For this review, take the finished solid that the model builds, in its own axes (mm). A direction names the side the tool comes from. Give positions to 0.01 mm unless a question says otherwise; leave off trailing zeros. Write each loop counter-clockwise with the first axis right and the second up, starting at its lowest first coordinate (ties: lowest second). Pieces come first, ordered by that corner, then holes.
Q1. We need section B-B (y = 122.5). Write out the cut boundary in (x, z), then the cut area to 3 significant figures.
Q2. For line 1 (X direction, y = 31, z = 0.75) (3 decimals); line 2 (X direction, y = 74, z = 6.25) (3 decimals); line 3 (X direction, y = 91, z = 0.5), list the stretches that pass through material, from the lowest coordinate up.
Q3. We need section A-A (y = 44.45). Write out the cut boundary in (x, z) (3 decimals).
Q4. Insertion check: P1, Ø3, axis at y = 33, z = 3, coming from the +X side; P2, Ø3, axis at x = 83, z = 3.5, coming from the -Y side; P3, Ø1.9, axis at y = 24.5, z = 4.5, coming from the +X side. Each pin has a flat end and moves straight along its axis. Give the tip position at first contact, or say it passes through.
Q5. Machinability: for faces 1 (the flat face through (-2, -12, 6.35)), 2 (the flat face through (38.1, 5, 3)), 3 (the flat face through (51, 28.448, 3)), which of the approach directions +Z, -Z, +X, -X, +Y, -Y give a long, thin tool a straight path to every point of the face, cutting with its end or side? Answer none if there is none.
Q6. Mouldability with a two-part tool opening along X and no side actions: class faces 4 (the flat face through (-2, -12, 0)), 5 (the cylindrical face through (-5.04, -82.45, 3.13)), 6 (the flat face through (-38.1, 5, 3)) as released by +X, released by -X, zero draft, split by the parting line, or undercut.
Q7. We need section D-D (x = 27.5). Write out the cut boundary in (y, z), then the cut area to 3 significant figures.
Q8. We need section C-C (x = 0). Write out the cut boundary in (y, z).
```python
from build123d import *

# Parameters (mm, degrees)
BOSS_EXTRUDE1_DEPTH = 6.35
CUT_EXTRUDE1_REACH  = 210.789
SKETCH2_R           = 1.3335
SKETCH2_W           = 24.765
SKETCH2_H           = 71.755
CUT_EXTRUDE2_REACH  = 210.789
SKETCH3_R           = 0.635
CUT_EXTRUDE3_DEPTH  = 209.788828163
FILLET1_START       = -1
FILLET1_DEPTH       = 8
FILLET1_2_DEPTH     = 6.35
SKETCH5_R           = 2.0828
CUT_EXTRUDE4_DEPTH  = 209.788828163


with BuildPart() as part:
    # Sketch1 → Boss-Extrude1 (new body)
    with BuildSketch(Plane.XY):
        with BuildLine():
            Line((-38.1, 92.71), (-38.1, 165.60027858))
            ThreePointArc((-38.1, 165.60027858), (0, -82.55), (38.1, 165.60027858))
            Line((38.1, 165.60027858), (38.1, 92.71))
            Line((38.1, 92.71), (38.1, -6.35))
            Line((38.1, -6.35), (-38.1, -6.35))
            Line((-38.1, -6.35), (-38.1, 92.71))
        make_face()
    extrude(amount=BOSS_EXTRUDE1_DEPTH)

    # Sketch2 → Cut-Extrude1 (cut, up to next)
    with BuildSketch(Plane(origin=(0, 0, 0), x_dir=(-1, 0, 0), z_dir=(0, 0, -1)), mode=Mode.PRIVATE) as cut_extrude1_sk1:
        with Locations((61.7855, 12.5095)):
            Circle(SKETCH2_R)
    cut_extrude1_tool1 = extrude(cut_extrude1_sk1.sketch, amount=-CUT_EXTRUDE1_REACH, mode=Mode.PRIVATE) & part.part
    # Sketch2 → Cut-Extrude1 (cut, up to next)
    with BuildSketch(Plane(origin=(0, 0, 0), x_dir=(-1, 0, 0), z_dir=(0, 0, -1)), mode=Mode.PRIVATE) as cut_extrude1_sk2:
        with Locations((61.7855, 84.6455)):
            Circle(SKETCH2_R)
    cut_extrude1_tool2 = extrude(cut_extrude1_sk2.sketch, amount=-CUT_EXTRUDE1_REACH, mode=Mode.PRIVATE) & part.part
    # Sketch2 → Cut-Extrude1 (cut, up to next)
    with BuildSketch(Plane(origin=(0, 0, 0), x_dir=(-1, 0, 0), z_dir=(0, 0, -1)), mode=Mode.PRIVATE) as cut_extrude1_sk3:
        with Locations((89.9795, 84.6455)):
            Circle(SKETCH2_R)
    cut_extrude1_tool3 = extrude(cut_extrude1_sk3.sketch, amount=-CUT_EXTRUDE1_REACH, mode=Mode.PRIVATE) & part.part
    # Sketch2 → Cut-Extrude1 (cut, up to next)
    with BuildSketch(Plane(origin=(0, 0, 0), x_dir=(-1, 0, 0), z_dir=(0, 0, -1)), mode=Mode.PRIVATE) as cut_extrude1_sk4:
        with Locations((89.9795, 12.5095)):
            Circle(SKETCH2_R)
    cut_extrude1_tool4 = extrude(cut_extrude1_sk4.sketch, amount=-CUT_EXTRUDE1_REACH, mode=Mode.PRIVATE) & part.part
    # Sketch2 → Cut-Extrude1 (cut, up to next)
    with BuildSketch(Plane(origin=(0, 0, 0), x_dir=(-1, 0, 0), z_dir=(0, 0, -1)), mode=Mode.PRIVATE) as cut_extrude1_sk5:
        with Locations((75.8825, 48.5775)):
            Rectangle(SKETCH2_W, SKETCH2_H)
    cut_extrude1_tool5 = extrude(cut_extrude1_sk5.sketch, amount=-CUT_EXTRUDE1_REACH, mode=Mode.PRIVATE) & part.part
    add(cut_extrude1_tool1.solids().sort_by_distance((-61.7855, 12.5095, 0))[0], mode=Mode.SUBTRACT)
    add(cut_extrude1_tool2.solids().sort_by_distance((-61.7855, 84.6455, 0))[0], mode=Mode.SUBTRACT)
    add(cut_extrude1_tool3.solids().sort_by_distance((-89.9795, 84.6455, 0))[0], mode=Mode.SUBTRACT)
    add(cut_extrude1_tool4.solids().sort_by_distance((-89.9795, 12.5095, 0))[0], mode=Mode.SUBTRACT)
    add(cut_extrude1_tool5.solids().sort_by_distance((-75.8825, 48.5775, 0))[0], mode=Mode.SUBTRACT)

    # Sketch3 → Cut-Extrude2 (cut, up to next)
    with BuildSketch(Plane.XY.offset(6.35), mode=Mode.PRIVATE) as cut_extrude2_sk1:
        with Locations((-66.04, 6.35)):
            Circle(SKETCH3_R)
    cut_extrude2_tool1 = extrude(cut_extrude2_sk1.sketch, amount=-CUT_EXTRUDE2_REACH, mode=Mode.PRIVATE) & part.part
    # Sketch3 → Cut-Extrude2 (cut, up to next)
    with BuildSketch(Plane.XY.offset(6.35), mode=Mode.PRIVATE) as cut_extrude2_sk2:
        with Locations((-71.628, 6.35)):
            Circle(SKETCH3_R)
    cut_extrude2_tool2 = extrude(cut_extrude2_sk2.sketch, amount=-CUT_EXTRUDE2_REACH, mode=Mode.PRIVATE) & part.part
    # Sketch3 → Cut-Extrude2 (cut, up to next)
    with BuildSketch(Plane.XY.offset(6.35), mode=Mode.PRIVATE) as cut_extrude2_sk3:
        with Locations((-80.137, 6.35)):
            Circle(SKETCH3_R)
    cut_extrude2_tool3 = extrude(cut_extrude2_sk3.sketch, amount=-CUT_EXTRUDE2_REACH, mode=Mode.PRIVATE) & part.part
    # Sketch3 → Cut-Extrude2 (cut, up to next)
    with BuildSketch(Plane.XY.offset(6.35), mode=Mode.PRIVATE) as cut_extrude2_sk4:
        with Locations((-85.725, 6.35)):
            Circle(SKETCH3_R)
    cut_extrude2_tool4 = extrude(cut_extrude2_sk4.sketch, amount=-CUT_EXTRUDE2_REACH, mode=Mode.PRIVATE) & part.part
    # Sketch3 → Cut-Extrude2 (cut, up to next)
    with BuildSketch(Plane.XY.offset(6.35), mode=Mode.PRIVATE) as cut_extrude2_sk5:
        with Locations((-73.0885, 90.805)):
            Circle(SKETCH3_R)
    cut_extrude2_tool5 = extrude(cut_extrude2_sk5.sketch, amount=-CUT_EXTRUDE2_REACH, mode=Mode.PRIVATE) & part.part
    # Sketch3 → Cut-Extrude2 (cut, up to next)
    with BuildSketch(Plane.XY.offset(6.35), mode=Mode.PRIVATE) as cut_extrude2_sk6:
        with Locations((-78.6765, 90.805)):
            Circle(SKETCH3_R)
    cut_extrude2_tool6 = extrude(cut_extrude2_sk6.sketch, amount=-CUT_EXTRUDE2_REACH, mode=Mode.PRIVATE) & part.part
    add(cut_extrude2_tool1.solids().sort_by_distance((-66.04, 6.35, 6.35))[0], mode=Mode.SUBTRACT)
    add(cut_extrude2_tool2.solids().sort_by_distance((-71.628, 6.35, 6.35))[0], mode=Mode.SUBTRACT)
    add(cut_extrude2_tool3.solids().sort_by_distance((-80.137, 6.35, 6.35))[0], mode=Mode.SUBTRACT)
    add(cut_extrude2_tool4.solids().sort_by_distance((-85.725, 6.35, 6.35))[0], mode=Mode.SUBTRACT)
    add(cut_extrude2_tool5.solids().sort_by_distance((-73.0885, 90.805, 6.35))[0], mode=Mode.SUBTRACT)
    add(cut_extrude2_tool6.solids().sort_by_distance((-78.6765, 90.805, 6.35))[0], mode=Mode.SUBTRACT)

    # Sketch4 → Cut-Extrude3 (cut, through all)
    with BuildSketch(Plane.XY.offset(6.35)):
        Polygon((-48.26, 72.898), (-48.26, 53.848), (-58.1, 53.848), (-58.1, 28.448), (-43.18, 28.448), (-43.18, 19.558), (-38.1, 19.558), (-38.1, 72.898), align=None)
        Polygon((43.18, 28.448), (58.1, 28.448), (58.1, 53.848), (48.26, 53.848), (48.26, 72.898), (38.1, 72.898), (38.1, 19.558), (43.18, 19.558), align=None)
    extrude(amount=-CUT_EXTRUDE3_DEPTH, mode=Mode.SUBTRACT)

    # Fillet1: read off the stored shape, not the designer's step
    # Fillet1 outline → Fillet1 (cut)
    with BuildSketch(Plane.XY.offset(FILLET1_START)):
        with BuildLine():
            Line((38.1, 72.898), (40.64, 72.898))
            ThreePointArc((40.64, 72.898), (38.843948776, 73.641948776), (38.1, 75.438))
            Line((38.1, 75.438), (38.1, 72.898))
        make_face()
        with BuildLine():
            Line((48.26, 53.848), (50.8, 53.848))
            ThreePointArc((50.8, 53.848), (49.003948776, 54.591948776), (48.26, 56.388))
            Line((48.26, 56.388), (48.26, 53.848))
        make_face()
        with BuildLine():
            Line((43.18, 28.448), (43.18, 25.908))
            ThreePointArc((43.18, 25.908), (43.923948776, 27.704051224), (45.72, 28.448))
            Line((45.72, 28.448), (43.18, 28.448))
        make_face()
        with BuildLine():
            ThreePointArc((38.1, 17.018), (38.843948776, 18.814051224), (40.64, 19.558))
            Line((40.64, 19.558), (38.1, 19.558))
            Line((38.1, 19.558), (38.1, 17.018))
        make_face()
        with BuildLine():
            Line((-38.1, 19.558), (-40.64, 19.558))
            ThreePointArc((-40.64, 19.558), (-38.843948776, 18.814051224), (-38.1, 17.018))
            Line((-38.1, 17.018), (-38.1, 19.558))
        make_face()
        with BuildLine():
            ThreePointArc((-38.1, 75.438), (-38.843948776, 73.641948776), (-40.64, 72.898))
            Line((-40.64, 72.898), (-38.1, 72.898))
            Line((-38.1, 72.898), (-38.1, 75.438))
        make_face()
        with BuildLine():
            ThreePointArc((-48.26, 56.388), (-49.003948776, 54.591948776), (-50.8, 53.848))
            Line((-50.8, 53.848), (-48.26, 53.848))
            Line((-48.26, 53.848), (-48.26, 56.388))
        make_face()
        with BuildLine():
            ThreePointArc((-45.72, 28.448), (-43.923948776, 27.704051224), (-43.18, 25.908))
            Line((-43.18, 25.908), (-43.18, 28.448))
            Line((-43.18, 28.448), (-45.72, 28.448))
        make_face()
    extrude(amount=FILLET1_DEPTH, mode=Mode.SUBTRACT)

    # Fillet1 2 outline → Fillet1 2 (add)
    with BuildSketch(Plane.XY):
        with BuildLine():
            Line((43.18, 19.558), (43.18, 22.098))
            ThreePointArc((43.18, 22.098), (42.436051224, 20.301948776), (40.64, 19.558))
            Line((40.64, 19.558), (43.18, 19.558))
        make_face()
        with BuildLine():
            ThreePointArc((45.72, 72.898), (47.516051224, 72.154051224), (48.26, 70.358))
            Line((48.26, 70.358), (48.26, 72.898))
            Line((48.26, 72.898), (45.72, 72.898))
        make_face()
        with BuildLine():
            ThreePointArc((55.56, 53.848), (57.356051224, 53.104051224), (58.1, 51.308))
            Line((58.1, 51.308), (58.1, 53.848))
            Line((58.1, 53.848), (55.56, 53.848))
        make_face()
        with BuildLine():
            ThreePointArc((58.1, 30.988), (57.356051224, 29.191948776), (55.56, 28.448))
            Line((55.56, 28.448), (58.1, 28.448))
            Line((58.1, 28.448), (58.1, 30.988))
        make_face()
        with BuildLine():
            Line((-43.18, 19.558), (-40.64, 19.558))
            ThreePointArc((-40.64, 19.558), (-42.436051224, 20.301948776), (-43.18, 22.098))
            Line((-43.18, 22.098), (-43.18, 19.558))
        make_face()
        with BuildLine():
            Line((-48.26, 72.898), (-48.26, 70.358))
            ThreePointArc((-48.26, 70.358), (-47.516051224, 72.154051224), (-45.72, 72.898))
            Line((-45.72, 72.898), (-48.26, 72.898))
        make_face()
        with BuildLine():
            Line((-58.1, 53.848), (-58.1, 51.308))
            ThreePointArc((-58.1, 51.308), (-57.356051224, 53.104051224), (-55.56, 53.848))
            Line((-55.56, 53.848), (-58.1, 53.848))
        make_face()
        with BuildLine():
            Line((-58.1, 28.448), (-55.56, 28.448))
            ThreePointArc((-55.56, 28.448), (-57.356051224, 29.191948776), (-58.1, 30.988))
            Line((-58.1, 30.988), (-58.1, 28.448))
        make_face()
    extrude(amount=FILLET1_2_DEPTH)

    # Sketch5 → Cut-Extrude4 (cut, through all)
    with BuildSketch(Plane.XY.offset(6.35)):
        with Locations((-45.085, 80.645)):
            Circle(SKETCH5_R)
        with Locations(Location((45.085, 80.645, 0), (0, 0, 180))):
            Circle(SKETCH5_R)
        with Locations((45.085, 15.875)):
            Circle(SKETCH5_R)
        with Locations(Location((-45.085, 15.875, 0), (0, 0, 180))):
            Circle(SKETCH5_R)
        with Locations((-45.085, 93.6625)):
            Circle(SKETCH5_R)
        with Locations(Location((45.085, 93.6625, 0), (0, 0, 180))):
            Circle(SKETCH5_R)
        with Locations((45.085, 2.8575)):
            Circle(SKETCH5_R)
        with Locations(Location((-45.085, 2.8575, 0), (0, 0, 180))):
            Circle(SKETCH5_R)
    extrude(amount=-CUT_EXTRUDE4_DEPTH, mode=Mode.SUBTRACT)


solid = part.part
```
Computed:
1. outline: (-100.19, 0) - (-38.1, 0) - (-38.1, 6.35) - (-100.19, 6.35) - close; (38.1, 0) - (100.19, 0) - (100.19, 6.35) - (38.1, 6.35) - close
1. area: 788 mm2
2. line 1: x = -126.286 to -88.265, -63.5 to -58.1, 58.1 to 126.286
2. line 2: x = -123.514 to -88.265, -63.5 to -38.546, 38.546 to 123.514
2. line 3: x = -118.16 to -79.28, -78.07 to -73.69, -72.48 to -38.1, 38.1 to 118.16
3. outline: (-127, 0) - (-88.265, 0) - (-88.265, 6.35) - (-127, 6.35) - close; (-63.5, 0) - (-58.1, 0) - (-58.1, 6.35) - (-63.5, 6.35) - close; (58.1, 0) - (127, 0) - (127, 6.35) - (58.1, 6.35) - close
4. P1: stops at x = 126.61
4. P2: stops at y = -52.95
4. P3: stops at x = 125.57
5. face 1: +Z, +X, -X, +Y, -Y
5. face 2: +Z, -Z, +Y
5. face 3: +Z, -Z
6. face 4: zero draft
6. face 5: split by the parting line
6. face 6: undercut
7. outline: (-79.54, 0) - (-6.35, 0) - (-6.35, 6.35) - (-79.54, 6.35) - close
7. area: 465 mm2
8. outline: (-82.55, 0) - (-6.35, 0) - (-6.35, 6.35) - (-82.55, 6.35) - close
